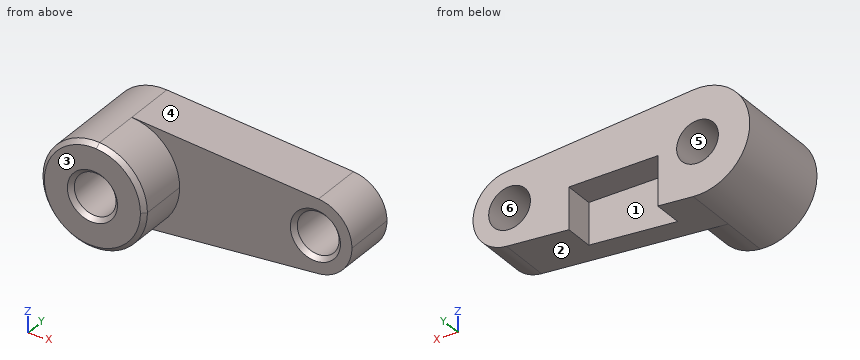
from build123d import *

# Parameters (mm, degrees)
F0_R     = 10
F1_DEPTH = 25
F2_DEPTH = 50
F3_SIZE  = 2
F4_W     = 42.542353
F4_H     = 60.176491
F5_DEPTH = 25


with BuildPart() as f1:
    # F0 (on Front) → F1 (new body)
    with BuildSketch(Plane.XZ):
        with BuildLine():
            ThreePointArc((2.083333, -24.913043), (18.399502, -16.92508), (25, 0))
            ThreePointArc((25, 0), (18.399502, 16.92508), (2.083333, 24.913043))
            ThreePointArc((2.083333, 24.913043), (-25, 0), (2.083333, -24.913043))
        make_face()
        Circle(F0_R, mode=Mode.SUBTRACT)
        with BuildLine():
            ThreePointArc((2.083333, 24.913043), (18.399502, 16.92508), (25, 0))
            ThreePointArc((25, 0), (18.399502, -16.92508), (2.083333, -24.913043))
            Line((2.083333, -24.913043), (91.458333, -17.43913))
            ThreePointArc((91.458333, -17.43913), (72.5, 0), (91.458333, 17.43913))
            Line((91.458333, 17.43913), (2.083333, 24.913043))
        make_face()
        with BuildLine():
            ThreePointArc((107.5, 0), (102.879651, 11.847556), (91.458333, 17.43913))
            ThreePointArc((91.458333, 17.43913), (72.5, 0), (91.458333, -17.43913))
            ThreePointArc((91.458333, -17.43913), (102.879651, -11.847556), (107.5, 0))
        make_face()
        with Locations((90, 0)):
            Circle(F0_R, mode=Mode.SUBTRACT)
    extrude(amount=F1_DEPTH)

    # F0 (on Front) → F2 (join)
    with BuildSketch(Plane.XZ):
        with BuildLine():
            ThreePointArc((2.083333, -24.913043), (18.399502, -16.92508), (25, 0))
            ThreePointArc((25, 0), (18.399502, 16.92508), (2.083333, 24.913043))
            ThreePointArc((2.083333, 24.913043), (-25, 0), (2.083333, -24.913043))
        make_face()
        Circle(F0_R, mode=Mode.SUBTRACT)
    extrude(amount=F2_DEPTH)

    # F3
    f3_edges = [f1.edges().sort_by_distance(p)[0] for p in [
        (-2.083333, -50, 24.913043),
        (-10, -50, 0),
        (80, -25, 0),
    ]]
    chamfer(f3_edges, length=F3_SIZE)

    # F4 (on Top) → F5 (cut)
    with BuildSketch(Plane.XY):
        with Locations((40.295548, 15.942938)):
            Rectangle(F4_W, F4_H)
    extrude(amount=-F5_DEPTH, mode=Mode.SUBTRACT)


solid = f1.part
Check sheet for the modelled part. Datum: model origin and axes. Units: mm. Face numbers are marked on the shaded views. A direction names the side the tool comes from. Round coordinates to 2 decimals unless told otherwise and drop trailing zeros. Loops run counter-clockwise (first coordinate to the right, second up) from the corner with the lowest first, then second, coordinate; pieces in that order, holes last. Notation, with made-up numbers: M 30.5,-25.75 L 86.5,-25.75 A16 ccw 86.5,-18.75 Z; hole C 56,27.25 d11. An arc over 180 degrees is marked long. One line per question, with ' | ' between items. Start each with the question number.
Item 1: Section check B-B (y = -6). Record the boundary of the cut face in (x, z).
Item 2: Gauge pin test, flat ends, axial feed: pin 1 Ø5 at (y, z) = (-37, -13.5) entering from -X; pin 2 Ø4 at (y, z) = (-40.5, -11.5) entering from +X; pin 3 Ø3 at (x, z) = (77.5, -1.5) entering from +Y; pin 4 Ø6 at (x, z) = (70, 4.5) entering from -Y. Record the tip position at first contact, or that the pin passes through.
Item 3: Scan lines: probe 1 along X at (y, z) = (-1.5, 0.5) (1 decimal); probe 2 along X at (y, z) = (-13.5, 6); probe 3 along Z at (x, y) = (90, -9.5). Record each from-to range of solid material in increasing order.
Item 4: Section check D-D (x = 90). Record the boundary of the cut face in (y, z).
Item 5: Section check C-C (y = -29). Record the boundary of the cut face in (x, z).
Item 6: Section check A-A (x = 0). Record the boundary of the cut face in (y, z), and give its area (3 significant figures).
Item 7: Release check for a two-part mould opening along Z. For the marked faces 3, 4, 5 and 6 record: released by +Z, released by -Z, zero draft, split by the parting line, or undercut.
Item 8: Set-up check for the marked faces 1 and 2: record each of +Z, -Z, +X, -X, +Y, -Y from which the full face is reachable in a straight line by a thin tool's end or side.
Worked out:
1) outline: M 2.08,-24.91 L 19.02,-23.5 L 19.02,0 L 61.57,0 L 61.57,-19.94 L 91.46,-17.44 A17.5 ccw 91.46,17.44 L 2.08,24.91 A25 ccw long Z; hole C 0,0 d20; hole C 90,0 d20
2) pin 1: x = -22.45 | pin 2: x = 23.12 | pin 3: y = 0 | pin 4: y = -25
3) probe 1: -25 to -10, 10 to 80, 100 to 107.5 | probe 2: -24.27 to -8, 8 to 82, 98 to 106.44 | probe 3: -17.56 to -10, 10 to 17.56
4) outline: M -25,-17.56 L 0,-17.56 L 0,-10 L -23,-10 L -25,-12 Z; M -25,12 L -23,10 L 0,10 L 0,17.56 L -25,17.56 Z
5) outline: M 2.08,-24.91 A25 ccw 25,0 A25 ccw 2.08,24.91 A25 ccw long Z; hole C 0,0 d20
6) outline: M -50,-23 L -48,-25 L 0,-25 L 0,-10 L -48,-10 L -50,-12 Z; M -50,12 L -48,10 L 0,10 L 0,25 L -48,25 L -50,23 Z | area: 1,490 mm^2
7) face 3: zero draft | face 4: released by +Z | face 5: undercut | face 6: undercut
8) face 1: -Z, +Y | face 2: -Z, +X, +Y, -Y
